Part model, mm, in its own coordinate system. A direction names the side the tool comes from. Coordinates: 2 decimals unless noted, no trailing zeros. Loops run counter-clockwise (first coordinate to the right, second up) from the corner with the lowest first, then second, coordinate; pieces in that order, holes last. Notation, with made-up numbers: M 34,-18.5 L 38,-18.5 A14 cw 38,-1.5 Z; hole C 3.5,28.5 d2. An arc over 180 degrees is marked long. Use a Markdown table: item, result. Add a question column.
1) Wall check: probe 1 along X at (y, z) = (0.4, -12.5); probe 2 along Z at (x, y) = (17.5, 0.4); probe 3 along Y at (x, z) = (10, -4.5). Give the ranges that are in metal, low to high. Write a range as from..to.
2) Band-saw the part on C-C (x = 36.5). List the corners of the cut face in (y, z).
3) Tool access for faces 1 (the flat face through (2, 2, -13)), 2 (the flat face through (20.5, 2, -12)), 3 (the flat face through (27, 2, -9)), 4 (the flat face through (2, 2, -2)): list every direction of +Z, -Z, +X, -X, +Y, -Y with a clear straight run to the whole face (end or side of a thin tool).
4) Band-saw the part on B-B (y = 0.4). List the corners of the cut face in (x, z).
5) Pin check, flat tips, straight feed: pin 1 Ø4.5 at (x, z) = (20, -5) entering from +Y; pin 2 Ø1.5 at (y, z) = (3, -9) entering from +X; pin 3 Ø2 at (x, z) = (17.5, -12.5) entering from -Y; pin 4 Ø1.5 at (x, y) = (28.5, 3.5) entering from +Z. Stop position of each tip, or through.
6) Band-saw the part on A-A (z = -12.5). List the corners of the cut face in (x, y).
7) Band-saw the part on D-D (x = 25.5). List the corners of the cut face in (y, z), plus the area to 3 significant figures.
8) Pull direction X, two halves, no side cores. Call faces 5 (the cylindrical face through (37.85, 0.49, -11.47)), 6 (the flat face through (2, 4, -8)), 7 (the flat face through (33.5, 2, -12)): released by +X, released by -X, zero draft, split by the parting line, or undercut.
from build123d import *

# Parameters (mm, degrees)
SKETCH1_W            = 39
SKETCH1_H            = 15
BOSS_EXTRUDE1_DEPTH  = 1
M3_CLEARANCE_HOLE1_D = 3.4
SKETCH4_W            = 13
SKETCH4_H            = 6
BOSS_EXTRUDE2_DEPTH  = 3
SKETCH5_W            = 5
SKETCH5_H            = 11
BOSS_EXTRUDE3_DEPTH  = 3


with BuildPart() as part:
    # Sketch1 → Boss-Extrude1 (new body)
    with BuildSketch(Plane(origin=(0, 0, 0), x_dir=(1, 0, 0), z_dir=(0, 1, 0))):
        with Locations((19.5, 7.5)):
            Rectangle(SKETCH1_W, SKETCH1_H)
    extrude(amount=BOSS_EXTRUDE1_DEPTH)

    # M3 Clearance Hole1 (through all)
    with Locations(Plane(origin=(0, 1, 0), x_dir=(1, 0, 0), z_dir=(0, 1, 0))):
        with Locations((36.5, 12.5), (17.5, 12.5)):
            Hole(M3_CLEARANCE_HOLE1_D / 2)

    # Sketch4 → Boss-Extrude2 (add)
    with BuildSketch(Plane(origin=(0, 1, 0), x_dir=(1, 0, 0), z_dir=(0, 1, 0))):
        with Locations((27, 12)):
            Rectangle(SKETCH4_W, SKETCH4_H)
    extrude(amount=BOSS_EXTRUDE2_DEPTH)

    # Sketch5 → Boss-Extrude3 (add)
    with BuildSketch(Plane(origin=(0, 1, 0), x_dir=(1, 0, 0), z_dir=(0, 1, 0))):
        with Locations((2.5, 7.5)):
            Rectangle(SKETCH5_W, SKETCH5_H)
    extrude(amount=BOSS_EXTRUDE3_DEPTH)


solid = part.part
Entries:
| question | item | result |
|---|---|---|
| 1 | probe 1 | 0..15.8, 19.2..34.8, 38.2..39 |
| 1 | probe 2 | -15..-14.2, -10.8..0 |
| 1 | probe 3 | 0..1 |
| 2 | outline | M 0,-15 L 1,-15 L 1,-14.2 L 0,-14.2 Z; M 0,-10.8 L 1,-10.8 L 1,0 L 0,0 Z |
| 3 | face 1 | -Z, -X, +Y |
| 3 | face 2 | +Z, -Z, +Y |
| 3 | face 3 | +Z, +X, +Y |
| 3 | face 4 | +Z, +X, -X, +Y |
| 4 | outline | M 0,-15 L 39,-15 L 39,0 L 0,0 Z; hole C 17.5,-12.5 d3.4; hole C 36.5,-12.5 d3.4 |
| 5 | pin 1 | y = 1 |
| 5 | pin 2 | x = 33.5 |
| 5 | pin 3 | through |
| 5 | pin 4 | z = -9 |
| 6 | outline | M 0,0 L 15.8,0 L 15.8,1 L 5,1 L 5,4 L 0,4 Z; M 19.2,0 L 34.8,0 L 34.8,1 L 33.5,1 L 33.5,4 L 20.5,4 L 20.5,1 L 19.2,1 Z; M 38.2,0 L 39,0 L 39,1 L 38.2,1 Z |
| 7 | outline | M 0,-15 L 4,-15 L 4,-9 L 1,-9 L 1,0 L 0,0 Z |
| 7 | area | 33.0 mm2 |
| 8 | face 5 | undercut |
| 8 | face 6 | zero draft |
| 8 | face 7 | released by +X |
